Part model, mm, in its own coordinate system. A direction names the side the tool comes from. Coordinates: 2 decimals unless noted, no trailing zeros. Loops run counter-clockwise (first coordinate to the right, second up) from the corner with the lowest first, then second, coordinate; pieces in that order, holes last. Notation, with made-up numbers: (-17, -2) -> (0, -2) arc R19 ccw to (0, 19) -> close; hole circle Ø1 at (10, -23.75). An arc over 180 degrees is marked (long way). Use one line per item in the form item = value. Start each with the question number.
(1) Drill centre lines: L1, parallel to X at y = 11, z = 0.7; L2, parallel to Y at x = 17, z = 1.6; L3, parallel to X at y = 18.5, z = 0.7. Where is each one in solid material? Low to high. Write a range as [from, to].
(2) Band-saw the part on C-C on z = 1.1. Give the cut face in (x, y).
(3) Pin check, flat tips, straight feed: P1, Ø0.5, axis at x = 32.5, z = 1, coming from the +Y side; P2, Ø0.5, axis at y = 18.5, z = 1.5, coming from the +X side. Stop position of each tip, or through.
(4) Band-saw the part on A-A on x = 6. Give the cut face in (y, z), then the cut area to 3 significant figures.
(5) 3-axis set-ups, long thin cutter, end or side, ignore diameter. For faces 1 (the flat face through (18.542, 13, 1)), 2 (the flat face through (3.81, 3, 1)), 3 (the flat face through (36.906, 15, 1)), 4 (the flat face through (0, 17, 1)): which of +Z, -Z, +X, -X, +Y, -Y reach the whole face in a straight line?
(6) Band-saw the part on D-D on y = 20.75. Give the cut face in (x, z).
(7) Band-saw the part on B-B on y = 8.5. Give the cut face in (x, z), then the cut area to 3 significant figures.
(8) Mould opens along X. For faces 5 (the flat face through (38, 22.53, 1)), 6 (the flat face through (-1.803, 8, 1)), 7 (the flat face through (2.54, 13, 1)) say: +X half, -X half, draft (parallel to the pull), parting line (faces both ways), or undercut.
```python
from build123d import *

# Parameters (mm, degrees)
BOSS_EXTRUDE1_DEPTH = 1.8034
SKETCH2_W           = 18.542
SKETCH2_H           = 2.8702
BOSS_EXTRUDE2_DEPTH = 1.8034


with BuildPart() as part:
    # Sketch1 → Boss-Extrude1 (new body)
    with BuildSketch(Plane.XY):
        Polygon((-1.8034, 12.0396), (0, 12.0396), (0, 19.6596), (2.54, 19.6596), (2.54, 6.2738), (18.542, 6.2738), (18.542, 22.5298), (21.4122, 22.5298), (21.4122, 6.7818), (36.9062, 6.7818), (36.9062, 22.5298), (39.3446, 22.5298), (39.3446, 6.7818), (54.8386, 6.7818), (54.8386, 22.5298), (56.134, 22.5298), (56.134, 12.0396), (57.9374, 12.0396), (57.9374, 4.7244), (52.324, 4.7244), (52.324, 1.5494), (3.81, 1.5494), (3.81, 4.7244), (-1.8034, 4.7244), align=None)
    extrude(amount=BOSS_EXTRUDE1_DEPTH)

    # Sketch2 → Boss-Extrude2 (add)
    with BuildSketch(Plane.XY.offset(1.8034)):
        with Locations((9.271, 21.0947)):
            Rectangle(SKETCH2_W, SKETCH2_H)
    extrude(amount=-BOSS_EXTRUDE2_DEPTH)


solid = part.part
```
A:
q1.L1 = [-1.8, 2.54], [18.54, 21.41], [36.91, 39.34], [54.84, 57.94]
q1.L2 = [1.55, 6.27], [19.66, 22.53]
q1.L3 = [0, 2.54], [18.54, 21.41], [36.91, 39.34], [54.84, 56.13]
q2.outline = (-1.8, 4.72) -> (3.81, 4.72) -> (3.81, 1.55) -> (52.32, 1.55) -> (52.32, 4.72) -> (57.94, 4.72) -> (57.94, 12.04) -> (56.13, 12.04) -> (56.13, 22.53) -> (54.84, 22.53) -> (54.84, 6.78) -> (39.34, 6.78) -> (39.34, 22.53) -> (36.91, 22.53) -> (36.91, 6.78) -> (21.41, 6.78) -> (21.41, 22.53) -> (0, 22.53) -> (0, 12.04) -> (-1.8, 12.04) -> close; hole (2.54, 6.27) -> (18.54, 6.27) -> (18.54, 19.66) -> (2.54, 19.66) -> close
q3.P1 = 6.78
q3.P2 = 56.13
q4.outline = (1.55, 0) -> (6.27, 0) -> (6.27, 1.8) -> (1.55, 1.8) -> close; (19.66, 0) -> (22.53, 0) -> (22.53, 1.8) -> (19.66, 1.8) -> close
q4.area = 13.7 mm²
q5.face_1 = +Z, -Z
q5.face_2 = +Z, -Z, -X, -Y
q5.face_3 = +Z, -Z, +Y
q5.face_4 = +Z, -Z, -X, +Y
q6.outline = (0, 0) -> (21.41, 0) -> (21.41, 1.8) -> (0, 1.8) -> close; (36.91, 0) -> (39.34, 0) -> (39.34, 1.8) -> (36.91, 1.8) -> close; (54.84, 0) -> (56.13, 0) -> (56.13, 1.8) -> (54.84, 1.8) -> close
q7.outline = (-1.8, 0) -> (2.54, 0) -> (2.54, 1.8) -> (-1.8, 1.8) -> close; (18.54, 0) -> (21.41, 0) -> (21.41, 1.8) -> (18.54, 1.8) -> close; (36.91, 0) -> (39.34, 0) -> (39.34, 1.8) -> (36.91, 1.8) -> close; (54.84, 0) -> (57.94, 0) -> (57.94, 1.8) -> (54.84, 1.8) -> close
q7.area = 23.0 mm²
q8.face_5 = draft
q8.face_6 = -X half
q8.face_7 = undercut
